Can you work these out from the drawing? Everything is in mm from the part's minimum corner. Round coordinates to 2 decimals unless told otherwise and drop trailing zeros. Write each loop counter-clockwise with the first axis right and the second up, starting at its lowest first coordinate (ties: lowest second). Pieces come first, ordered by that corner, then holes. Notation, with made-up numbers: (-11, -3.75) -> (10, -3.75) arc R18 ccw to (10, 0.25) -> close; hole circle Ø8 at (78.25, 58.25). An arc over 180 degrees is marked (long way). Answer as CSV lines item,"result". Start each with the question number.
Q1. If I drill on line 1 (Y direction, x = 48.7, z = 8); line 2 (X direction, y = 8, z = 66.5); line 3 (Y direction, x = 48.6, z = 15), over which ranges is the centre line in solid material (lowest first)? Write a range as [from, to].
Q2. If we mould it in two halves opening along Y, with no side actions, what happens to the marked faces 1, 2, 3 and 4? For each: pulls with the +Y half, pulls with the -Y half, needs draft (parallel to the pull), parting line crosses it, or undercut.
Q3. Will these pins go through, and if not, where does the flat tip stop? pin 1 Ø8 at (y, z) = (8, 40) entering from -X; pin 2 Ø1.5 at (x, z) = (44, 19.5) entering from +Y.
Q4. Imagine slicing it at A-A on y = 15. Please give me the cut outline in (x, z), and give its area (3 significant figures).
Q5. Imagine slicing it at B-B on x = 20.5. Please give me the cut outline in (y, z).
Q6. Imagine slicing it at C-C on z = 43. Please give me the cut outline in (x, y).
Q7. Imagine slicing it at D-D on y = 37. Please give me the cut outline in (x, z), and give its area (3 significant figures).
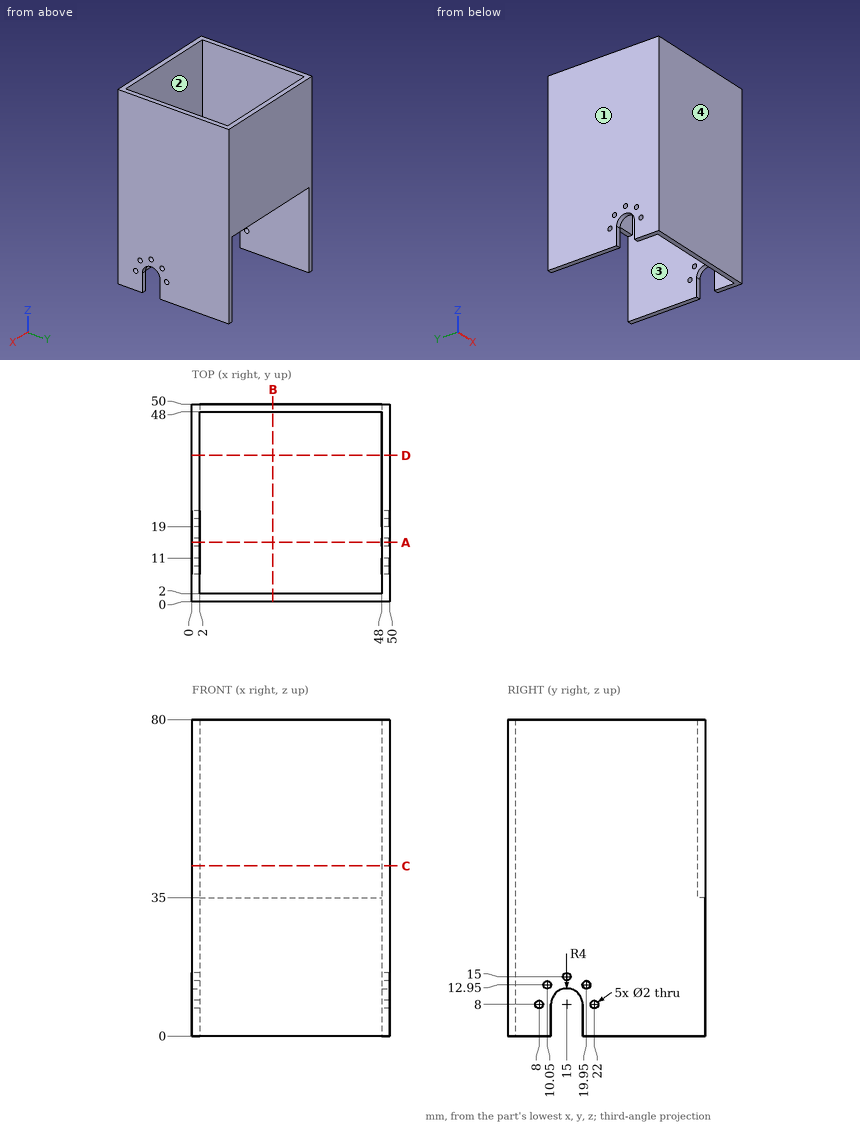
Checks:
1,line 1,"[0, 7], [9, 11], [19, 21], [23, 50]"
1,line 2,"[0, 2], [48, 50]"
1,line 3,"[0, 14], [16, 50]"
2,face 1,"needs draft"
2,face 2,"undercut"
2,face 3,"undercut"
2,face 4,"pulls with the -Y half"
3,pin 1,"x = 0"
3,pin 2,"y = 2"
4,outline,"(0, 12) -> (2, 12) -> (2, 14) -> (0, 14) -> close; (0, 16) -> (2, 16) -> (2, 80) -> (0, 80) -> close; (48, 12) -> (50, 12) -> (50, 14) -> (48, 14) -> close; (48, 16) -> (50, 16) -> (50, 80) -> (48, 80) -> close"
4,area,"264 mm^2"
5,outline,"(0, 0) -> (2, 0) -> (2, 80) -> (0, 80) -> close; (48, 35) -> (50, 35) -> (50, 80) -> (48, 80) -> close"
6,outline,"(0, 0) -> (50, 0) -> (50, 50) -> (0, 50) -> close; hole (2, 2) -> (48, 2) -> (48, 48) -> (2, 48) -> close"
7,outline,"(0, 0) -> (2, 0) -> (2, 80) -> (0, 80) -> close; (48, 0) -> (50, 0) -> (50, 80) -> (48, 80) -> close"
7,area,"320 mm^2"
